```python
from build123d import *

# Parameters (mm, degrees)
SKETCH2_W           = 45
SKETCH2_H           = 10
BOSS_EXTRUDE1_DEPTH = 40
SKETCH4_W           = 45
SKETCH4_H           = 10
BOSS_EXTRUDE2_DEPTH = 10
SKETCH8_W           = 45
SKETCH8_H           = 10
BOSS_EXTRUDE3_DEPTH = 20
SKETCH9_R           = 1.45
CUT_EXTRUDE2_DEPTH  = 20
SKETCH10_W          = 45
SKETCH10_H          = 0.626165357
CUT_EXTRUDE3_DEPTH  = 2


with BuildPart() as part:
    # Sketch2 → Boss-Extrude1 (new body)
    with BuildSketch(Plane(origin=(0, 0, 0), x_dir=(1, 0, 0), z_dir=(0, 1, 0))):
        Rectangle(SKETCH2_W, SKETCH2_H)
    extrude(amount=BOSS_EXTRUDE1_DEPTH)

    # Sketch4 → Boss-Extrude2 (add)
    with BuildSketch(Plane(origin=(0, 40, 0), x_dir=(1, 0, 0), z_dir=(0, 1, 0))):
        Rectangle(SKETCH4_W, SKETCH4_H)
    extrude(amount=BOSS_EXTRUDE2_DEPTH)

    # Sketch8 → Boss-Extrude3 (add)
    with BuildSketch(Plane.XZ):
        Rectangle(SKETCH8_W, SKETCH8_H)
    extrude(amount=BOSS_EXTRUDE3_DEPTH)

    # Sketch9 → Cut-Extrude2 (cut)
    with BuildSketch(Plane.XY.offset(5)):
        with Locations((19.5, 11.5)):
            Circle(SKETCH9_R)
        with Locations((-19.5, 11.5)):
            Circle(SKETCH9_R)
    extrude(amount=-CUT_EXTRUDE2_DEPTH, mode=Mode.SUBTRACT)

    # Sketch10 → Cut-Extrude3 (cut)
    with BuildSketch(Plane.XY.offset(5)):
        with Locations((0, 22.984410254)):
            Rectangle(SKETCH10_W, SKETCH10_H)
    extrude(amount=-CUT_EXTRUDE3_DEPTH, mode=Mode.SUBTRACT)


solid = part.part
```
Check sheet for the modelled part. Datum: model origin and axes. Units: mm. A direction names the side the tool comes from. Give positions to 0.01 mm unless a question says otherwise; leave off trailing zeros. Loops run counter-clockwise (first coordinate to the right, second up) from the corner with the lowest first, then second, coordinate; pieces in that order, holes last. Notation, with made-up numbers: M 37,-27 L 89,-27 A23 ccw 89,-17 Z; hole C 35.25,86 d6. An arc over 180 degrees is marked long. Answer in a Markdown table with one row per item.
1) Cross-section at A-A (x = -19.5). Enter the section's corners in (y, z).
Solutions:
| item | result |
|---|---|
| outline | M -20,-5 L 10.05,-5 L 10.05,5 L -20,5 Z; M 12.95,-5 L 50,-5 L 50,5 L 23.3,5 L 23.3,3 L 22.67,3 L 22.67,5 L 12.95,5 Z |
2) Mould release check, pull along Y, two halves, no side actions. Record for faces 1 (the face through (0, 50, 0)), 2 (the face through (-22.5, 15, 0)), 3 (the face through (0, 22.671, 4)): released by +Y, released by -Y, zero draft, split by the parting line, or undercut.
Solutions:
| item | result |
|---|---|
| face 1 | released by +Y |
| face 2 | zero draft |
| face 3 | undercut |
3) Tool access check on faces 4 (the face through (20.839, 10.945, 0.07)), 5 (the face through (0, 23.297, 4)). Record the directions out of +Z, -Z, +X, -X, +Y, -Y that give a thin tool (end or side, any length) a straight path to the whole face; none if there is none.
Solutions:
| item | result |
|---|---|
| face 4 | +Z, -Z |
| face 5 | +Z, +X, -X |
4) Cross-section at B-B (y = 11.5). Enter the section's corners in (x, z), plus the area to 3 significant figures.
Solutions:
| item | result |
|---|---|
| outline | M -22.5,-5 L -20.95,-5 L -20.95,5 L -22.5,5 Z; M -18.05,-5 L 18.05,-5 L 18.05,5 L -18.05,5 Z; M 20.95,-5 L 22.5,-5 L 22.5,5 L 20.95,5 Z |
| area | 392 mm^2 |
5) Thickness scan on line 1 (Y direction, x = 19.5, z = 0.5). Record the ranges inside material, lowest first.
Solutions:
| item | result |
|---|---|
| line 1 | y = -20 to 10.05, 12.95 to 50 |
6) Depth check by flat-ended pin: pin 1 (2.5 mm diameter, centred on x = -19.5, y = 11.5, fed in from -Z); pin 2 (0.5 mm diameter, centred on x = 7, y = 23, fed in from +Z). Enter the tip coordinate at first touch or a pass-through.
Solutions:
| item | result |
|---|---|
| pin 1 | passes through |
| pin 2 | stops at z = 3 |
